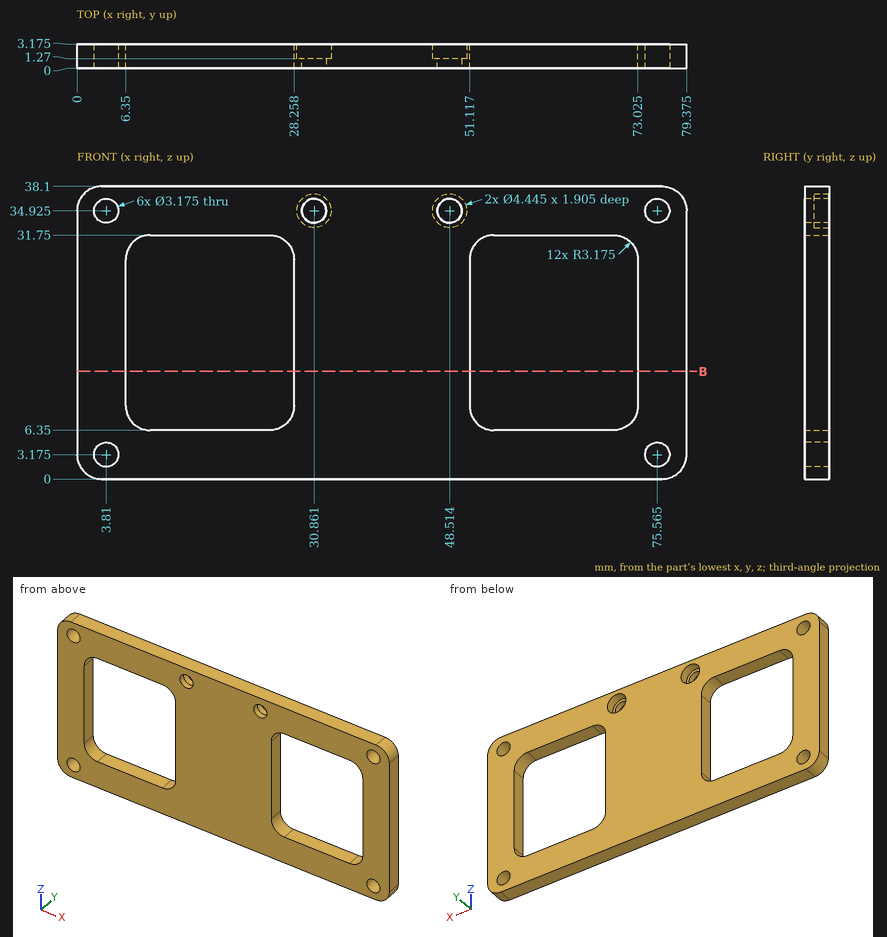
Geometry check sheet. Reference: drawing and pictorial views, mm from the part's lowest x, y, z. Give positions to 0.01 mm unless a question says otherwise; leave off trailing zeros. Answer in a Markdown table with one row per item.
1) Gauge pin test, flat ends, axial feed: P1, Ø4, axis at x = 3.81, z = 3.175, coming from the +Y side (1 decimal); P2, Ø2, axis at x = 49, z = 34.5, coming from the +Y side. Record the tip position at first contact, or that the pin passes through.
Filled sheet:
| item | result |
|---|---|
| P1 | stops at y = 3.2 |
| P2 | stops at y = 1.27 |
2) Cross-section at B-B, the plane z = 14. Count the separate pieces of the cut face and the enclosed holes in it, plus the area to 3 significant figures.
Filled sheet:
| item | result |
|---|---|
| separate pieces | 3 |
| enclosed holes | 0 |
| area | 113 mm2 |
3) Thickness scan on L1, parallel to Z at x = 3.81, y = 1.5; L2, parallel to X at y = 2.4, z = 29 (1 decimal); L3, parallel to Z at x = 62.5, y = 1.2. Record the ranges inside material, lowest first. Write a range as [from, to].
Filled sheet:
| item | result |
|---|---|
| L1 | z = [0, 1.59], [4.76, 33.34], [36.51, 38.1] |
| L2 | x = [0, 6.4], [28.2, 51.1], [73, 79.4] |
| L3 | z = [0, 6.35], [31.75, 38.1] |
